```python
from build123d import *

# Parameters (mm, degrees)
F2_R     = 15
F3_DEPTH = 25


with BuildPart() as f1:
    # F0 (on Front) → F1 (revolve)
    with BuildSketch(Plane.XZ):
        with BuildLine():
            Line((0, 4), (0, 0))
            Line((0, 0), (72.2, 0))
            Line((72.2, 0), (76.2, 0))
            Line((76.2, 0), (76.2, 4))
            Line((76.2, 4), (76.2, 24))
            Line((76.2, 24), (72.2, 24))
            Line((72.2, 24), (72.2, 8))
            ThreePointArc((72.2, 8), (71.028427, 5.171573), (68.2, 4))
            Line((68.2, 4), (0, 4))
        make_face()
    revolve(axis=Axis((0, 0, 2), (0, 0, 1)))

    # F2 (on face) → F3 (cut)
    with BuildSketch(Plane.XY.offset(4)):
        Circle(F2_R)
    extrude(amount=-F3_DEPTH, mode=Mode.SUBTRACT)


solid = f1.part
```
Source: CAD feature listing. Evaluate the final solid. Frame: model axes, mm. A direction names the side the tool comes from. Round coordinates to 2 decimals unless told otherwise and drop trailing zeros. Write each loop counter-clockwise with the first axis right and the second up, starting at its lowest first coordinate (ties: lowest second). Pieces come first, ordered by that corner, then holes. Notation, with made-up numbers: M 47,-24.5 L 57,-24.5 A9 cw 57,-12.5 Z; hole C 26.25,-2 d9. An arc over 180 degrees is marked long. Answer as a JSON object with one key per item and string values. Group by question number.
(1) Section query C-C on z = 20.75. Output: boundary loops of the cut face in (x, y).
(2) Section query A-A on y = 0. Output: boundary loops of the cut face in (x, z), then the cut area to 3 significant figures.
(3) Reachability of faces 4 (the flat face through (-1, 16, 4)), 5 (the cylindrical face through (-14.985, 0.66, 2.028)) from +Z, -Z, +X, -X, +Y, -Y: full face, straight path, thin tool, end or side. Return the list, or none.
(4) Ray query, line 1 (Y direction, x = 0, z = 12.75); line 2 (Y direction, x = 0, z = 2.25); line 3 (X direction, y = -56, z = 22). Return the intervals inside material, ascending. Write a range as [from, to].
(5) Mould query, pull axis X, two halves, no side actions, for faces 1 (the cylindrical face through (-15.652, -70.483, 15.888)), 2 (the flat face through (-16, 1, 0)), 3 (the cylindrical face through (-60.47, -46.367, 12.168)). Classes: +X half, -X half, draft (parallel to the pull), parting line (faces both ways), or undercut.
(6) First-contact query: pin 1 (6 mm diameter, centred on x = 52.5, z = 18.5, fed in from -Y); pin 2 (6 mm diameter, centred on y = -56.5, z = 3.5, fed in from +X); pin 3 (2 mm diameter, centred on x = 14, z = 8.5, fed in from -Y). Flat tips, straight axial feed; report the tip coordinate or a pass-through.
Computed values:
{
 "1": {"outline": "C 0,0 d152.4; hole C 0,0 d144.4"},
 "2": {"outline": "M -76.2,0 L -15,0 L -15,4 L -68.2,4 A4 cw -72.2,8 L -72.2,24 L -76.2,24 Z; M 15,0 L 76.2,0 L 76.2,24 L 72.2,24 L 72.2,8 A4 cw 68.2,4 L 15,4 Z", "area": "656 mm^2"},
 "3": {"face 4": "+Z", "face 5": "+Z, -Z"},
 "4": {"line 1": "[-76.2, -72.2], [72.2, 76.2]", "line 2": "[-76.2, -15], [15, 76.2]", "line 3": "[-51.68, -45.57], [45.57, 51.68]"},
 "5": {"face 1": "undercut", "face 2": "draft", "face 3": "parting line"},
 "6": {"pin 1": "y = -57.93", "pin 2": "x = 54.26", "pin 3": "y = -75.08"}
}
